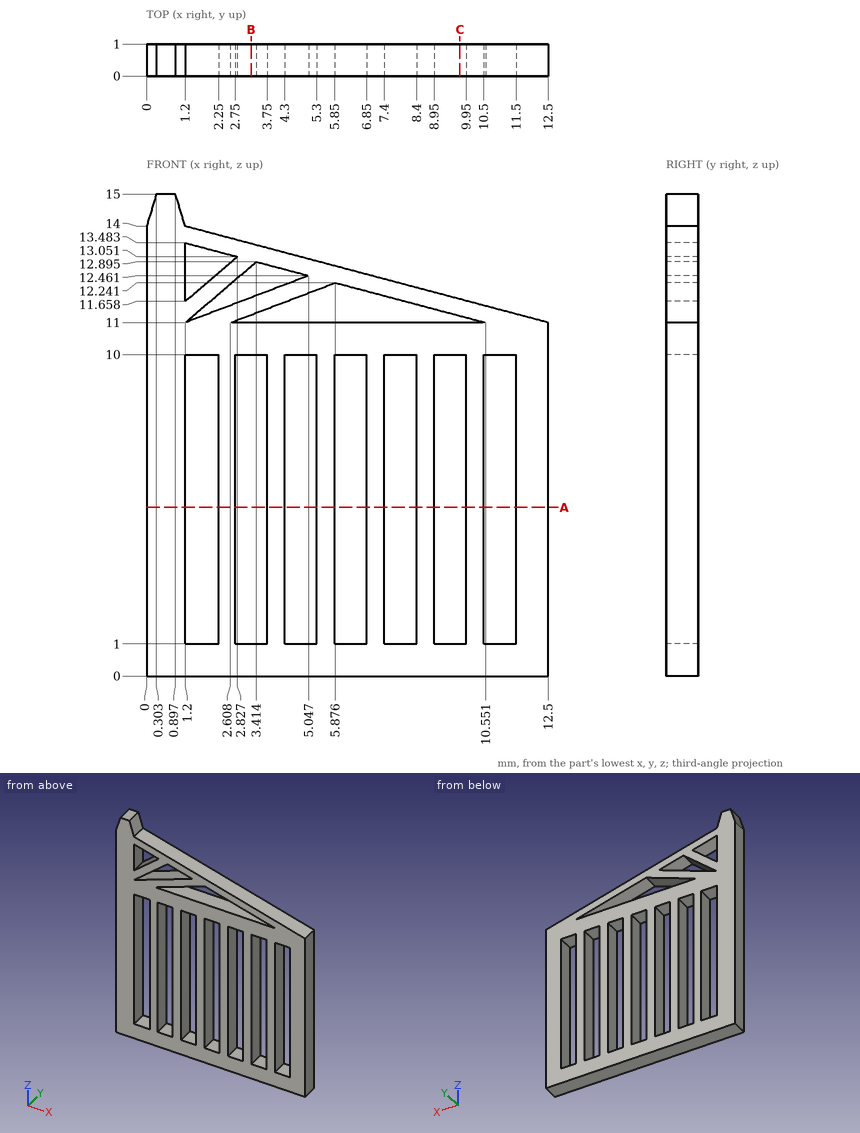
Source: three-view drawing plus pictorial views. Frame: mm from the lowest corner of the part. Round coordinates to 2 decimals unless told otherwise and drop trailing zeros. Write each loop counter-clockwise with the first axis right and the second up, starting at its lowest first coordinate (ties: lowest second). Pieces come first, ordered by that corner, then holes. Notation, with made-up numbers: M 13.25,-12 L 29.25,-12 A34 ccw 29.25,25 Z; hole C 3.25,-16.75 d1. An arc over 180 degrees is marked long. Use CSV: the item, a comma, the result in double quotes. Start each with the question number.
Q1. Line query: line 1 (Z direction, x = 8, y = 0.2) (1 decimal); line 2 (Z direction, x = 2, y = 0.7) (1 decimal); line 3 (Z direction, x = 6, y = 0.85) (1 decimal). Output: solid intervals per line, ascending. Write a range as from..to.
Q2. Cut plane B-B on x = 3.25. Output: boundary loops of the cut face in (y, z) (1 decimal).
Q3. Cut plane C-C on x = 9.75. Output: boundary loops of the cut face in (y, z).
Q4. Cut plane A-A on z = 5.25. Count the separate pieces of the cut face and the enclosed holes in it.
Q5. First-contact query: P1, Ø0.5, axis at x = 3, y = 0.5, coming from the +Z side; P2, Ø0.5, axis at x = 11, y = 0.5, coming from the +Z side (1 decimal); P3, Ø0.5, axis at x = 7.5, y = 0.5, coming from the +Z side. Flat tips, straight axial feed; report the tip coordinate or a pass-through.
Results found:
1,line 1,"0..1, 10..11, 11.7..12.2"
1,line 2,"0..1, 10..11.3, 11.7..12.3, 13.3..13.8"
1,line 3,"0..1, 10..11, 12.2..12.7"
2,outline,"M 0,0 L 1,0 L 1,1 L 0,1 Z; M 0,10 L 1,10 L 1,11 L 0,11 Z; M 0,11.2 L 1,11.2 L 1,11.8 L 0,11.8 Z; M 0,12.8 L 1,12.8 L 1,13.5 L 0,13.5 Z"
3,outline,"M 0,0 L 1,0 L 1,1 L 0,1 Z; M 0,10 L 1,10 L 1,11 L 0,11 Z; M 0,11.21 L 1,11.21 L 1,11.73 L 0,11.73 Z"
4,separate pieces,"8"
4,enclosed holes,"0"
5,P1,"z = 13.59"
5,P2,"z = 11.5"
5,P3,"z = 12.39"
